Design review of the part shown in the three views and the two pictorial views. Dimensions are in mm from the part's minimum x, y and z. A direction names the side the tool comes from. Round coordinates to 2 decimals unless told otherwise and drop trailing zeros. Order: outer loops, then holes, each group sorted by start corner. A loop starts at its lowest first (then second) coordinate and runs counter-clockwise, first axis right, second up.
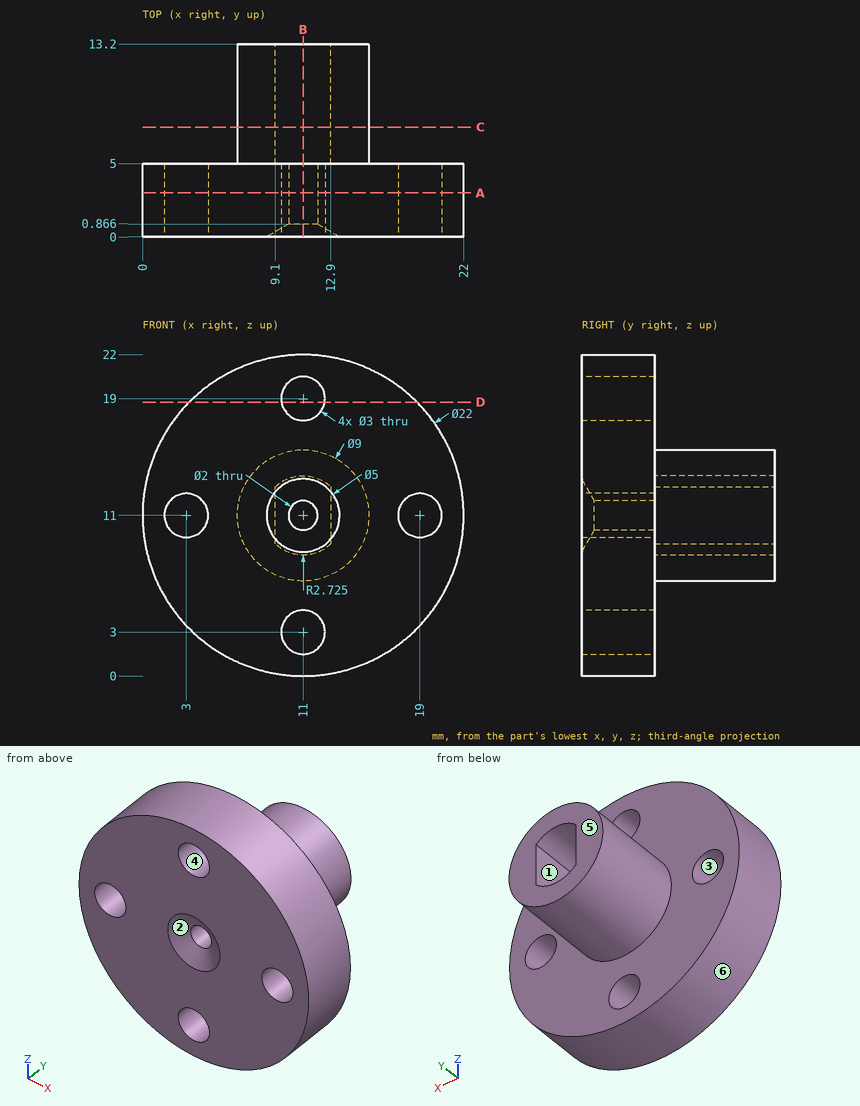
(1) To check wall thickness, follow probe 1 along X at (y, z) = (2.55, 11); probe 2 along Y at (x, z) = (19, 17.5); probe 3 along Z at (x, y) = (12.75, 10.5). State the ranges of each line that lie inside material, in increasing order.
Data:
probe 1: x = 0 to 1.5, 4.5 to 10, 12 to 17.5, 20.5 to 22
probe 2: y = 0 to 5
probe 3: z = 6.85 to 8.91, 13.09 to 15.15
(2) Draft analysis for pull direction X (two halves, no side actions). For the marked faces 3, 4, 5 and 6, state which applies: pulls with the +X half, pulls with the -X half, needs draft (parallel to the pull), parting line crosses it, or undercut.
Data:
face 3: undercut
face 4: undercut
face 5: needs draft
face 6: parting line crosses it
(3) For the marked faces 1 and 2, list the 3-axis set-ups (+Z, -Z, +X, -X, +Y, -Y) from which the entire face can be reached by the end or side of a thin tool; tool diameter is ignored.
Data:
face 1: +Y
face 2: -Y
(4) Consider section C-C (y = 7.5). Write out the cut boundary in (x, z) (3 decimals).
Data:
outline: circle Ø9 at (11, 11); hole (9.1, 9.047) arc R2.725 ccw to (12.9, 9.047) - (12.9, 12.953) arc R2.725 ccw to (9.1, 12.953) - close
(5) Insertion check: pin 1 (1.5 mm diameter, centred on y = 8.5, z = 5.5, fed in from -X); pin 2 (2 mm diameter, centred on y = 9.5, z = 11, fed in from -X); pin 3 (2 mm diameter, centred on y = 7.5, z = 10, fed in from +X); pin 4 (4 mm diameter, centred on x = 19.5, z = 11.5, fed in from +Y). Each pin has a flat end and moves straight along its axis. Give the tip position at first contact, or say it passes through.
Data:
pin 1: passes through
pin 2: stops at x = 6.5
pin 3: stops at x = 15.5
pin 4: stops at y = 5
(6) Consider section D-D (z = 18.75). Write out the cut boundary in (x, y), and give its area (3 significant figures).
Data:
outline: (3.19, 0) - (9.52, 0) - (9.52, 5) - (3.19, 5) - close; (12.48, 0) - (18.81, 0) - (18.81, 5) - (12.48, 5) - close
area: 63.3 mm2
(7) Consider section A-A (y = 3). Write out the cut boundary in (x, z), and give its area (3 significant figures).
Data:
outline: circle Ø22 at (11, 11); hole circle Ø3 at (3, 11); hole circle Ø3 at (11, 3); hole circle Ø3 at (11, 19); hole circle Ø2 at (11, 11); hole circle Ø3 at (19, 11)
area: 349 mm2
(8) Consider section B-B (x = 11). Write out the cut boundary in (y, z) (3 decimals), and give its area (3 significant figures).
Data:
outline: (0, 0) - (5, 0) - (5, 1.5) - (0, 1.5) - close; (0, 4.5) - (5, 4.5) - (5, 6.5) - (13.2, 6.5) - (13.2, 8.275) - (5, 8.275) - (5, 10) - (0.866, 10) - (0, 8.5) - close; (0, 13.5) - (0.866, 12) - (5, 12) - (5, 13.725) - (13.2, 13.725) - (13.2, 15.5) - (5, 15.5) - (5, 17.5) - (0, 17.5) - close; (0, 20.5) - (5, 20.5) - (5, 22) - (0, 22) - close
area: 97.8 mm2
